Design review of the part built by this model. Coordinates are the model's own, in mm. A direction names the side the tool comes from. Coordinates: 2 decimals unless noted, no trailing zeros. Write each loop counter-clockwise with the first axis right and the second up, starting at its lowest first coordinate (ties: lowest second). Pieces come first, ordered by that corner, then holes.
Q1. Insertion check: pin 1 (3 mm diameter, centred on y = 15.5, z = -15.5, fed in from -X); pin 2 (5 mm diameter, centred on y = 9, z = -28, fed in from +X). Each pin has a flat end and moves straight along its axis. Give the tip position at first contact, or say it passes through.
Q2. Machinability: for faces 1 (the flat face through (9, -5, -30)), 2 (the flat face through (6, 21.25, -9)), 3 (the flat face through (3, -12.75, -30)), which of the approach directions +Z, -Z, +X, -X, +Y, -Y give a long, thin tool a straight path to every point of the face, cutting with its end or side? Answer none if there is none.
Q3. Take a section at C-C (x = 11.25). Give the boundary of the cut face in (y, z), and give its area (3 significant figures).
Q4. Take a section at A-A (z = 15.5). Give the boundary of the cut face in (x, y).
Q5. Mouldability with a two-part tool opening along Z and no side actions: class faces 4 (the flat face through (12, 0, -16)), 5 (the cylindrical face through (2.96, 9.94, -25.75)), 6 (the flat face through (3, -7.25, -30)) as pulls with the +Z half, pulls with the -Z half, needs draft (parallel to the pull), parting line crosses it, or undercut.
Q6. Take a section at B-B (y = 0). Give the boundary of the cut face in (x, z).
Q7. For probe 1 along Y at (x, z) = (7, 15.5); probe 2 along Z at (x, y) = (8.75, -14); probe 3 along Y at (x, z) = (9, 14), list the stretches that pass through material, from the lowest coordinate up.
Q8. Take a section at D-D (z = 0). Give the boundary of the cut face in (x, y).
```python
from build123d import *

# Parameters (mm, degrees)
SKETCH2_W           = 61
SKETCH2_H           = 42.5
SKETCH2_R           = 11.5
SKETCH2_R_2         = 1.75
BOSS_EXTRUDE2_DEPTH = 12
CUT_EXTRUDE1_DEPTH  = 6


with BuildPart() as part:
    # Sketch2 → Boss-Extrude2 (new body)
    with BuildSketch(Plane(origin=(0, 0, 0), x_dir=(0, 0, -1), z_dir=(1, 0, 0))):
        with Locations((9.5, 0)):
            Rectangle(SKETCH2_W, SKETCH2_H)
        Circle(SKETCH2_R, mode=Mode.SUBTRACT)
        with Locations((-15.5, 15.5)):
            Circle(SKETCH2_R_2, mode=Mode.SUBTRACT)
        with Locations((15.5, -15.5)):
            Circle(SKETCH2_R_2, mode=Mode.SUBTRACT)
        with Locations((15.5, 15.5)):
            Circle(SKETCH2_R_2, mode=Mode.SUBTRACT)
        with Locations((-15.5, -15.5)):
            Circle(SKETCH2_R_2, mode=Mode.SUBTRACT)
        with BuildLine():
            Line((28.5, 12.75), (31.5, 12.75))
            ThreePointArc((31.5, 12.75), (34.25, 10), (31.5, 7.25))
            Line((31.5, 7.25), (28.5, 7.25))
            ThreePointArc((28.5, 7.25), (25.75, 10), (28.5, 12.75))
        make_face(mode=Mode.SUBTRACT)
        with BuildLine():
            Line((28.5, -12.75), (31.5, -12.75))
            ThreePointArc((31.5, -12.75), (34.25, -10), (31.5, -7.25))
            Line((31.5, -7.25), (28.5, -7.25))
            ThreePointArc((28.5, -7.25), (25.75, -10), (28.5, -12.75))
        make_face(mode=Mode.SUBTRACT)
    extrude(amount=BOSS_EXTRUDE2_DEPTH)

    # Sketch3 → Cut-Extrude1 (cut)
    with BuildSketch(Plane(origin=(12, 0, 0), x_dir=(0, 0, -1), z_dir=(1, 0, 0))):
        with BuildLine():
            Line((28.5, 15), (31.5, 15))
            ThreePointArc((31.5, 15), (36.5, 10), (31.5, 5))
            Line((31.5, 5), (28.5, 5))
            ThreePointArc((28.5, 5), (23.5, 10), (28.5, 15))
        make_face()
        with BuildLine():
            Line((28.5, -15), (31.5, -15))
            ThreePointArc((31.5, -15), (36.5, -10), (31.5, -5))
            Line((31.5, -5), (28.5, -5))
            ThreePointArc((28.5, -5), (23.5, -10), (28.5, -15))
        make_face()
    extrude(amount=-CUT_EXTRUDE1_DEPTH, mode=Mode.SUBTRACT)


solid = part.part
```
Response:
1. pin 1: passes through
1. pin 2: stops at x = 6
2. face 1: +X
2. face 2: +Z, -Z, +X, -X, +Y
2. face 3: +X, -X
3. outline: (-21.25, -40) - (21.25, -40) - (21.25, 21) - (-21.25, 21) - close; hole circle Ø3.5 at (-15.5, -15.5); hole circle Ø3.5 at (-15.5, 15.5); hole (-15, -31.5) arc R5 ccw to (-5, -31.5) - (-5, -28.5) arc R5 ccw to (-15, -28.5) - close; hole circle Ø23 at (0, 0); hole (5, -31.5) arc R5 ccw to (15, -31.5) - (15, -28.5) arc R5 ccw to (5, -28.5) - close; hole circle Ø3.5 at (15.5, -15.5); hole circle Ø3.5 at (15.5, 15.5)
3. area: 1,920 mm2
4. outline: (0, -21.25) - (12, -21.25) - (12, -17.25) - (0, -17.25) - close; (0, -13.75) - (12, -13.75) - (12, 13.75) - (0, 13.75) - close; (0, 17.25) - (12, 17.25) - (12, 21.25) - (0, 21.25) - close
5. face 4: needs draft
5. face 5: undercut
5. face 6: undercut
6. outline: (0, -40) - (12, -40) - (12, -11.5) - (0, -11.5) - close; (0, 11.5) - (12, 11.5) - (12, 21) - (0, 21) - close
7. probe 1: y = -21.25 to -17.25, -13.75 to 13.75, 17.25 to 21.25
7. probe 2: z = -40 to -34.5, -25.5 to -16.4, -14.6 to 14.6, 16.4 to 21
7. probe 3: y = -21.25 to -16.4, -14.6 to 14.6, 16.4 to 21.25
8. outline: (0, -21.25) - (12, -21.25) - (12, -11.5) - (0, -11.5) - close; (0, 11.5) - (12, 11.5) - (12, 21.25) - (0, 21.25) - close
